```python
from build123d import *

# Parameters (mm, degrees)
F0_R     = 1.6
F1_DEPTH = 2


# Not quite as in the source:
# - ends of sketch curves that miss each other by under 0.0002 mm in the source are joined


with BuildPart() as f1:
    # F0 (on Top) → F1 (new body)
    with BuildSketch(Plane.XY):
        with BuildLine():
            ThreePointArc((9.4743104318, 0.2374556452), (11.0743104318, 1.8374556452), (12.6743104318, 0.2374556452))
            Line((12.6743104318, 0.2374556452), (22.0509076786, 0.2374556452))
            Line((22.0509076786, 0.2374556452), (31.3863246398, 0.2374556452))
            ThreePointArc((31.3863246398, 0.2374556452), (32.9863104318, 1.8374556452), (34.5863104318, 0.2374556452))
            Line((34.5863104318, 0.2374556452), (36.9589188956, 0.2374556452))
            ThreePointArc((36.9589188956, 0.2374556452), (37.322944486, 1.4299580557), (38.4322782501, 1.9991287063))
            Line((38.4322782501, 1.9991287063), (39.8303104318, 10.0774704438))
            Line((39.8303104318, 10.0774704438), (39.8303104318, 25.8181473703))
            Line((39.8303104318, 25.8181473703), (38.0968938881, 34.5188772837))
            add(Edge.make_bspline(
                [(38.0968938881, 34.5188772837), (37.6683242364, 35.7597207754), (36.7252101224, 38.130874007), (34.7779775897, 39.0193902227), (33.5303104318, 39.4987425759)],
                knots=[0, 0, 0, 0, 0.51039131, 1, 1, 1, 1], degree=3))
            ThreePointArc((33.5303104318, 39.4987425759), (32.6165966127, 39.7845023129), (31.6957953827, 40.0465264824))
            ThreePointArc((31.6957953827, 40.0465264824), (31.3007464304, 40.007865889), (31.0303104318, 39.7173100649))
            Line((31.0303104318, 39.7173100649), (31.0303104318, 34.5188772837))
            Line((31.0303104318, 34.5188772837), (31.0303104318, 31.1867967248))
            Line((31.0303104318, 31.1867967248), (32.5903408229, 29.2609930038))
            Line((32.5903408229, 29.2609930038), (32.5903408229, 27.0907320082))
            Line((32.5903408229, 27.0907320082), (22.0303104318, 27.0907320082))
            Line((22.0303104318, 27.0907320082), (11.4702800406, 27.0907320082))
            Line((11.4702800406, 27.0907320082), (11.4702800406, 29.2609930038))
            Line((11.4702800406, 29.2609930038), (13.0303104318, 31.1867967248))
            Line((13.0303104318, 31.1867967248), (13.0303104318, 34.5188772837))
            Line((13.0303104318, 34.5188772837), (13.0303104318, 39.7173100649))
            ThreePointArc((13.0303104318, 39.7173100649), (12.7598744332, 40.007865889), (12.3648254809, 40.0465264824))
            ThreePointArc((12.3648254809, 40.0465264824), (11.4440242509, 39.7845023129), (10.5303104318, 39.4987425759))
            add(Edge.make_bspline(
                [(5.9637269754, 34.5188772837), (6.3922966272, 35.7597207754), (7.3354107411, 38.130874007), (9.2826432739, 39.0193902227), (10.5303104318, 39.4987425759)],
                knots=[0, 0, 0, 0, 0.51039131, 1, 1, 1, 1], degree=3))
            Line((5.9637269754, 34.5188772837), (4.2303104318, 25.8181473703))
            Line((4.2303104318, 25.8181473703), (4.2303104318, 10.0774704438))
            Line((4.2303104318, 10.0774704438), (5.6569326528, 1.8339249926))
            ThreePointArc((5.6569326528, 1.8339249926), (6.7190254428, 1.3306221238), (7.1506988404, 0.2374556452))
            Line((7.1506988404, 0.2374556452), (9.4743104318, 0.2374556452))
        make_face()
        Polygon((11.5445189413, 7.2601027762), (22.0303104318, 7.2601027762), (32.5161019223, 7.2601027762), (32.6645797236, 7.2601027762), (32.6645797236, 5.0898417806), (32.5161019223, 5.0898417806), (11.5445189413, 5.0898417806), (11.39604114, 5.0898417806), (11.39604114, 7.2601027762), align=None, mode=Mode.SUBTRACT)
        Polygon((18.7320070459, 17.286), (22.0303104318, 20.3086156398), (25.3286138177, 17.286), (22.0303104318, 13.222059235), align=None, mode=Mode.SUBTRACT)
        Polygon((8.1803104318, 15.401), (7.3303104318, 15.401), (7.3303104318, 21.601), (8.1803104318, 21.601), (9.0303104318, 21.601), (9.0303104318, 15.401), align=None, mode=Mode.SUBTRACT)
        with Locations((10.5303104318, 34.5188772837)):
            Circle(F0_R, mode=Mode.SUBTRACT)
        Polygon((35.0303104318, 15.401), (35.0303104318, 21.601), (35.8803104318, 21.601), (36.7303104318, 21.601), (36.7303104318, 15.401), (35.8803104318, 15.401), align=None, mode=Mode.SUBTRACT)
        with Locations((33.5303104318, 34.5188772837)):
            Circle(F0_R, mode=Mode.SUBTRACT)
    extrude(amount=F1_DEPTH)


solid = f1.part
```
Could you check a few things on this model? Use its own coordinates, in mm. A direction names the side the tool comes from. Coordinates: 2 decimals unless noted, no trailing zeros. Write each loop counter-clockwise with the first axis right and the second up, starting at its lowest first coordinate (ties: lowest second). Pieces come first, ordered by that corner, then holes. Notation, with made-up numbers: (61, 46.5) -> (101, 46.5) arc R11 ccw to (101, 55.5) -> close; hole circle Ø8 at (79.25, 50.5). An arc over 180 degrees is marked (long way). Write item = value, one per line. Start each with the question number.
(1) I want a section at B-B (y = 30). Please give me the cut outline in (x, z), plus the area to 3 significant figures.
(2) I need wall thicknesses on line 1 (Y direction, x = 24, z = 0.85); line 2 (Y direction, x = 21.5, z = 1.75); line 3 (Y direction, x = 30.5, z = 1.85). Which ranges of each line are inside material? Lowest first, please. Write a range as [from, to].
(3) We'd pull the mould along X, two halves only. Please class faces 1 (the face through (22, 0.237, 1)), 2 (the face through (32.951, 1.837, 0.986)), 3 (the face through (6.71, 1.34, 0.99)): released by +X, released by -X, zero draft, split by the parting line, or undercut.
(4) Will these pins go through, and if not, where does the flat tip stop? pin 1 (0.6 mm diameter, centred on y = 27.5, z = 0.5, fed in from +X) (3 decimals); pin 2 (1 mm diameter, centred on y = 32, z = 1, fed in from +X); pin 3 (0.6 mm diameter, centred on y = 28, z = 1, fed in from -X).
(5) I want a section at C-C (x = 20). Please give me the cut outline in (y, z).
(6) I want a section at A-A (x = 15.5). Please give me the cut outline in (y, z).
(7) Which directions (+Z, -Z, +X, -X, +Y, -Y) give clear straight access to the entire face, cutting with the end or side of a thin tool? Please do faces 4 (the face through (20.4, 15.23, 0.99)), 5 (the face through (8, 0.237, 1)).
(8) I want a section at D-D (z = 0.95). Give the number of separate pieces and of enclosed holes in the cut face, plus the area to 3 significant figures.
Result set:
q1.outline = (5.06, 0) -> (12.07, 0) -> (12.07, 2) -> (5.06, 2) -> close; (31.99, 0) -> (39, 0) -> (39, 2) -> (31.99, 2) -> close
q1.area = 28.0 mm2
q2.line_1 = [0.24, 5.09], [7.26, 15.65], [18.5, 27.09]
q2.line_2 = [0.24, 5.09], [7.26, 13.88], [19.82, 27.09]
q2.line_3 = [0.24, 5.09], [7.26, 27.09]
q3.face_1 = zero draft
q3.face_2 = undercut
q3.face_3 = released by -X
q4.pin_1 = 39.555
q4.pin_2 = 38.7
q4.pin_3 = 4.61
q5.outline = (0.24, 0) -> (5.09, 0) -> (5.09, 2) -> (0.24, 2) -> close; (7.26, 0) -> (15.72, 0) -> (15.72, 2) -> (7.26, 2) -> close; (18.45, 0) -> (27.09, 0) -> (27.09, 2) -> (18.45, 2) -> close
q6.outline = (0.24, 0) -> (5.09, 0) -> (5.09, 2) -> (0.24, 2) -> close; (7.26, 0) -> (27.09, 0) -> (27.09, 2) -> (7.26, 2) -> close
q7.face_4 = +Z, -Z
q7.face_5 = +Z, -Z, +X, -X, -Y
q8.separate_pieces = 1
q8.enclosed_holes = 6
q8.area = 985 mm2
